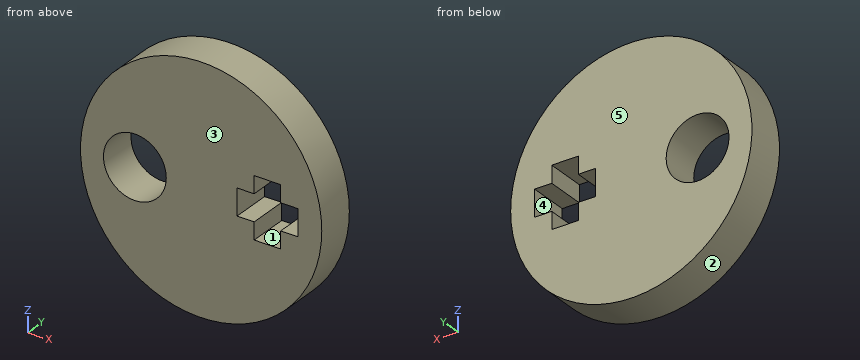
from build123d import *

# Parameters (mm, degrees)
SKETCH1_R           = 9.1
SKETCH1_R_2         = 2.37
BOSS_EXTRUDE1_DEPTH = 3


with BuildPart() as part:
    # Sketch1 → Boss-Extrude1 (new body)
    with BuildSketch(Plane(origin=(0, 0, 0), x_dir=(1, 0, 0), z_dir=(0, 1, 0))):
        Circle(SKETCH1_R)
        with Locations((-5, 0)):
            Circle(SKETCH1_R_2, mode=Mode.SUBTRACT)
        Polygon((7.291287847, -1), (6, -1), (6, -2.291287847), (4, -2.291287847), (4, -1), (2.708712153, -1), (2.708712153, 1), (4, 1), (4, 2.291287847), (6, 2.291287847), (6, 1), (7.291287847, 1), align=None, mode=Mode.SUBTRACT)
    extrude(amount=BOSS_EXTRUDE1_DEPTH)


solid = part.part
Can you work these out from the model? Positions are in its coordinate system, mm. Face numbers are marked on the shaded views. A direction names the side the tool comes from. Coordinates: 2 decimals unless noted, no trailing zeros. Write each loop counter-clockwise with the first axis right and the second up, starting at its lowest first coordinate (ties: lowest second). Pieces come first, ordered by that corner, then holes.
Q1. Imagine slicing it at A-A, the plane y = 2.4. List the corners of the cut face in (x, z) for me, plus the area to 3 significant figures.
Results found:
outline: circle Ø18.2 at (0, 0); hole circle Ø4.74 at (-5, 0); hole (2.71, -1) - (4, -1) - (4, -2.29) - (6, -2.29) - (6, -1) - (7.29, -1) - (7.29, 1) - (6, 1) - (6, 2.29) - (4, 2.29) - (4, 1) - (2.71, 1) - close
area: 228 mm2
Q2. Imagine slicing it at C-C, the plane x = 7. List the corners of the cut face in (y, z) for me.
Results found:
outline: (0, -5.81) - (3, -5.81) - (3, -1) - (0, -1) - close; (0, 1) - (3, 1) - (3, 5.81) - (0, 5.81) - close
Q3. Which directions (+Z, -Z, +X, -X, +Y, -Y) give clear straight access to the entire face, cutting with the end or side of a thin tool? Please do the marked faces 4 and 5.
Results found:
face 4: +Y, -Y
face 5: +Z, -Z, +X, -X, +Y
Q4. If we mould it in two halves opening along X, with no side actions, what happens to the marked faces 1, 2 and 3? For each: +X half, -X half, draft (parallel to the pull), parting line (faces both ways), or undercut.
Results found:
face 1: undercut
face 2: parting line
face 3: draft
Q5. For P1, Ø1.4, axis at y = 2, z = 2, coming from the +X side; P2, Ø0.6, axis at x = 6.5, y = 1.5, coming from the -Z side; P3, Ø1.5, axis at y = 1, z = -5, coming from the -X side, each with a flat end and sliding along its axis, tell me the tip position at first contact or that it passes through.
Results found:
P1: stops at x = 9.01
P2: stops at z = -6.66
P3: stops at x = -8.05
Q6. Please list where these lines run through material, in increasing order: L1, parallel to X at y = 1.5, z = 0; L2, parallel to Z at x = -5.25, y = 0.35; L3, parallel to Z at x = -3.75, y = 1.9.
Results found:
L1: x = -9.1 to -7.37, -2.63 to 2.71, 7.29 to 9.1
L2: z = -7.43 to -2.36, 2.36 to 7.43
L3: z = -8.29 to -2.01, 2.01 to 8.29
Q7. Imagine slicing it at D-D, the plane x = 3.75. List the corners of the cut face in (y, z) for me, plus the area to 3 significant figures.
Results found:
outline: (0, -8.29) - (3, -8.29) - (3, -1) - (0, -1) - close; (0, 1) - (3, 1) - (3, 8.29) - (0, 8.29) - close
area: 43.7 mm2
Q8. Imagine slicing it at B-B, the plane z = 0. List the corners of the cut face in (x, y) for me.
Results found:
outline: (-9.1, 0) - (-7.37, 0) - (-7.37, 3) - (-9.1, 3) - close; (-2.63, 0) - (2.71, 0) - (2.71, 3) - (-2.63, 3) - close; (7.29, 0) - (9.1, 0) - (9.1, 3) - (7.29, 3) - close
